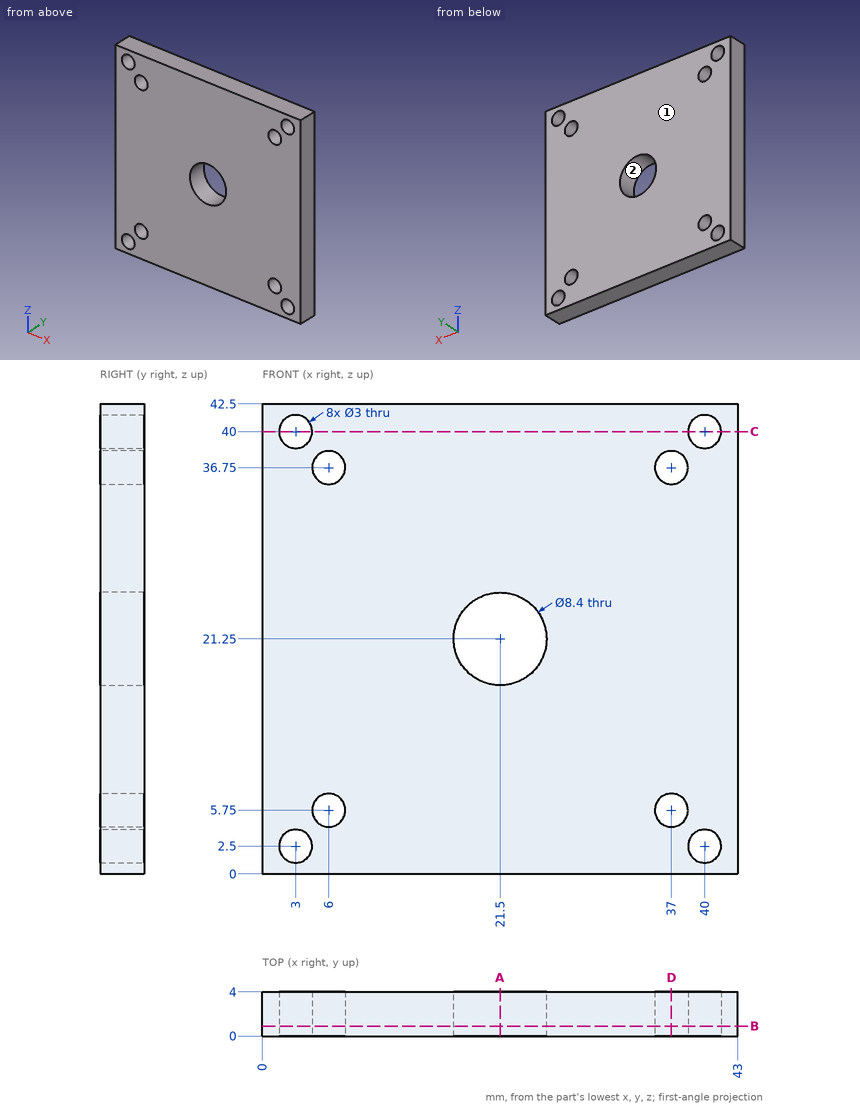
Job drawing, mm, ordinate dimensions from the low corner. One solid piece. Coordinates: 2 decimals unless noted, no trailing zeros. Write each loop counter-clockwise with the first axis right and the second up, starting at its lowest first coordinate (ties: lowest second). Pieces come first, ordered by that corner, then holes. Notation, with made-up numbers: M -33,41.5 L -29,41.5 A16 cw -29,54.5 Z; hole C -16,12.25 d4. An arc over 180 degrees is marked long. Answer as a JSON object with one key per item and string values. Group by question number.
1) Saw through at B-B (y = 0.9). Give the number of separate pieces and of enclosed holes in the cut face, plus the area to 3 significant figures.
2) Saw through at C-C (z = 40). Write the cut outline in (x, y).
3) Mould opens along Z. For the marked faces 1 and 2 say: +Z half, -Z half, draft (parallel to the pull), parting line (faces both ways), or undercut.
4) Wall check: line 1 (X direction, y = 2.05, z = 40); line 2 (X direction, y = 2.9, z = 36.75); line 3 (Z direction, x = 7, y = 3.25). Give the ranges that are in metal, low to high. Write a range as from..to.
5) Pin check, flat tip, straight feed: pin 1 Ø2.5 at (x, z) = (37, 5.75) entering from -Y. Stop position of the tip, or through.
6) Saw through at A-A (x = 21.5). Write the cut outline in (y, z), plus the area to 3 significant figures.
7) Saw through at D-D (x = 37). Write the cut outline in (y, z), plus the area to 3 significant figures.
Values follow:
{
 "1": {"separate pieces": "1", "enclosed holes": "9", "area": "1,720 mm2"},
 "2": {"outline": "M 0,0 L 1.5,0 L 1.5,4 L 0,4 Z; M 4.5,0 L 38.5,0 L 38.5,4 L 4.5,4 Z; M 41.5,0 L 43,0 L 43,4 L 41.5,4 Z"},
 "3": {"face 1": "draft", "face 2": "undercut"},
 "4": {"line 1": "x = 0..1.5, 4.5..38.5, 41.5..43", "line 2": "x = 0..4.5, 7.5..35.5, 38.5..43", "line 3": "z = 0..4.63, 6.87..35.63, 37.87..42.5"},
 "5": {"pin 1": "passes through"},
 "6": {"outline": "M 0,0 L 4,0 L 4,17.05 L 0,17.05 Z; M 0,25.45 L 4,25.45 L 4,42.5 L 0,42.5 Z", "area": "136 mm2"},
 "7": {"outline": "M 0,0 L 4,0 L 4,4.25 L 0,4.25 Z; M 0,7.25 L 4,7.25 L 4,35.25 L 0,35.25 Z; M 0,38.25 L 4,38.25 L 4,42.5 L 0,42.5 Z", "area": "146 mm2"}
}
